Verification items for the finished model (mm, model axes). A direction names the side the tool comes from. Give positions to 0.01 mm unless a question says otherwise; leave off trailing zeros. Loops run counter-clockwise (first coordinate to the right, second up) from the corner with the lowest first, then second, coordinate; pieces in that order, holes last. Notation, with made-up numbers: (15.5, 41.25) - (27.5, 41.25) arc R4 cw to (27.5, 46.25) - close; hole circle Ø6 at (2.25, 77.5). An arc over 180 degrees is marked (long way). One line per question, with ' | ' between items. Start each with the question number.
1. Depth check by flat-ended pin: pin 1 Ø1 at (x, y) = (-11, 0.5) entering from +Z; pin 2 Ø1.5 at (y, z) = (-14.5, -35) entering from -X; pin 3 Ø6 at (x, z) = (16.5, 67) entering from +Y. Enter the tip coordinate at first touch or a pass-through.
2. Thickness scan on line 1 along Z through (x, y) = (-8, -16); line 2 along Y through (x, z) = (0, 78); line 3 along X through (y, z) = (9, -10). Record the ranges inside material, lowest first. Write a range as from..to.
3. Mould release check, pull along Y, two halves, no side actions. Record for faces 1 (the face through (16, 15.82, 18.74)), 2 (the face through (0, -22.5, 19)), 3 (the face through (15.213, 4.791, -0.986)), 4 (the face through (22.5, 0, 19)): +Y half, -Y half, draft (parallel to the pull), parting line (faces both ways), or undercut.
4. Section check B-B, the plane z = 61. Enter the section's corners in (x, y).
5. Section check A-A, the plane x = 0. Enter the section's corners in (y, z), then the cut area to 3 significant figures.
6. Tool access check on faces 5 (the face through (0, 22.5, 19)), 6 (the face through (9, -9, 50)), 7 (the face through (9, -11, -2)). Record the directions out of +Z, -Z, +X, -X, +Y, -Y that give a thin tool (end or side, any length) a straight path to the whole face; none if there is none.
from build123d import *

# Parameters (mm, degrees)
SKETCH_1_R      = 15.95
SKETCH_1_R_2    = 14.05
EXTRUDE_1_DEPTH = 2
SKETCH_2_R      = 22.5
SKETCH_2_R_2    = 11
EXTRUDE_2_DEPTH = 50
SKETCH_3_R      = 21.05
EXTRUDE_3_DEPTH = 70
SKETCH_5_R      = 21.05
EXTRUDE_5_DEPTH = 40


with BuildPart() as part:
    # 스케치1 → 보스-돌출1 (new body)
    with BuildSketch(Plane.XY):
        Circle(SKETCH_1_R)
        Circle(SKETCH_1_R_2, mode=Mode.SUBTRACT)
    extrude(amount=-EXTRUDE_1_DEPTH)

    # 스케치2 → 보스-돌출2 (add)
    with BuildSketch(Plane.XY):
        Circle(SKETCH_2_R)
        Circle(SKETCH_2_R_2, mode=Mode.SUBTRACT)
    extrude(amount=EXTRUDE_2_DEPTH)

    # 스케치3 → 보스-돌출3 (add, symmetric)
    with BuildSketch(Plane.XY):
        Polygon((-9.319805153, -22.5), (9.319805153, -22.5), (22.5, -9.319805153), (22.5, 9.319805153), (9.319805153, 22.5), (-9.319805153, 22.5), (-22.5, 9.319805153), (-22.5, -9.319805153), align=None)
        Circle(SKETCH_3_R, mode=Mode.SUBTRACT)
    extrude(amount=EXTRUDE_3_DEPTH, both=True)

    # 스케치5 → 보스-돌출5 (add)
    with BuildSketch(Plane.XY.offset(70)):
        Polygon((-22.5, -9.319805153), (-9.319805153, -22.5), (9.319805153, -22.5), (22.5, -9.319805153), (22.5, 9.319805153), (9.319805153, 22.5), (-9.319805153, 22.5), (-22.5, 9.319805153), align=None)
        Circle(SKETCH_5_R, mode=Mode.SUBTRACT)
    extrude(amount=EXTRUDE_5_DEPTH)


solid = part.part
Results list:
1) pin 1: z = 50 | pin 2: x = -18.07 | pin 3: y = 18.32
2) line 1: 0..50 | line 2: -22.5..-21.05, 21.05..22.5 | line 3: -22.5..-19.03, 19.03..22.5
3) face 1: +Y half | face 2: -Y half | face 3: undercut | face 4: draft
4) outline: (-22.5, -9.32) - (-9.32, -22.5) - (9.32, -22.5) - (22.5, -9.32) - (22.5, 9.32) - (9.32, 22.5) - (-9.32, 22.5) - (-22.5, 9.32) - close; hole circle Ø42.1 at (0, 0)
5) outline: (-22.5, -70) - (-21.05, -70) - (-21.05, 0) - (-15.95, 0) - (-15.95, -2) - (-14.05, -2) - (-14.05, 0) - (-11, 0) - (-11, 50) - (-21.05, 50) - (-21.05, 110) - (-22.5, 110) - close; (11, 0) - (14.05, 0) - (14.05, -2) - (15.95, -2) - (15.95, 0) - (21.05, 0) - (21.05, -70) - (22.5, -70) - (22.5, 110) - (21.05, 110) - (21.05, 50) - (11, 50) - close | area: 1,530 mm²
6) face 5: +Z, -Z, +X, -X, +Y | face 6: +Z | face 7: -Z
